```python
from build123d import *

# Parameters (mm, degrees)
SKIZZE1_W                       = 61.8
SKIZZE1_H                       = 93.64
AUFSATZ_LINEAR_AUSTRAGEN1_DEPTH = 6
VERRUNDUNG1_R                   = 6
WANDUNG1_T                      = -1
SKIZZE2_W                       = 21.5
SKIZZE2_H                       = 9.5
SCHNITT_LINEAR_AUSTRAGEN1_DEPTH = 6
SKIZZE3_W                       = 22
SKIZZE3_H                       = 5
SCHNITT_LINEAR_AUSTRAGEN2_DEPTH = 6
SCHNITT_LINEAR_AUSTRAGEN4_DEPTH = 6
LINEARES_MUSTER1_COUNT          = 3
LINEARES_MUSTER1_PITCH          = 25


with BuildPart() as part:
    # Skizze1 → Aufsatz-Linear austragen1 (new body)
    with BuildSketch(Plane(origin=(0, 0, 0), x_dir=(0, 1, 0), z_dir=(0, 0, 1))):
        Rectangle(SKIZZE1_W, SKIZZE1_H)
    extrude(amount=AUFSATZ_LINEAR_AUSTRAGEN1_DEPTH)

    # Verrundung1
    verrundung1_edges = [part.edges().sort_by_distance(p)[0] for p in [
        (46.82, 30.9, 3),
        (46.82, -30.9, 3),
        (-46.82, -30.9, 3),
        (-46.82, 30.9, 3),
    ]]
    fillet(verrundung1_edges, radius=VERRUNDUNG1_R)

    # Wandung1
    wandung1_openings = [part.faces().sort_by_distance(p)[0] for p in [
        (0, 0, 6),
    ]]
    offset(amount=WANDUNG1_T, openings=wandung1_openings, kind=Kind.INTERSECTION)

    # Skizze2 → Schnitt-Linear austragen1 (cut)
    with BuildSketch(Plane.YZ.offset(46.82)):
        with Locations((0, 6)):
            Rectangle(SKIZZE2_W, SKIZZE2_H)
    extrude(amount=-SCHNITT_LINEAR_AUSTRAGEN1_DEPTH, mode=Mode.SUBTRACT)

    # Skizze3 → Schnitt-Linear austragen2 (cut)
    with BuildSketch(Plane.XZ.offset(30.9)):
        with Locations((-11.18, 3.5)):
            Rectangle(SKIZZE3_W, SKIZZE3_H)
    extrude(amount=-SCHNITT_LINEAR_AUSTRAGEN2_DEPTH, mode=Mode.SUBTRACT)

    # Skizze4 → Schnitt-Linear austragen4 (cut)
    with BuildSketch(Plane(origin=(0, 0, 0), x_dir=(1, 0, 0), z_dir=(0, 0, -1))):
        Polygon((-25.159745962, 25.45), (-33.82, 20.45), (-33.82, 10.45), (-25.159745962, 5.45), (-16.499491924, 10.45), (-16.499491924, 20.45), align=None)
        Polygon((-25.159745962, -4.35), (-33.82, -9.35), (-33.82, -19.35), (-25.159745962, -24.35), (-16.499491924, -19.35), (-16.499491924, -9.35), align=None)
    schnitt_linear_austragen4 = extrude(amount=-SCHNITT_LINEAR_AUSTRAGEN4_DEPTH, mode=Mode.SUBTRACT)

    # Lineares Muster1: Schnitt-Linear austragen4 ×3
    with Locations(*[(i * LINEARES_MUSTER1_PITCH, 0, 0) for i in range(1, LINEARES_MUSTER1_COUNT)]):
        add(schnitt_linear_austragen4, mode=Mode.SUBTRACT)


solid = part.part
```
Can you work these out from the model? Positions are in its coordinate system, mm. A direction names the side the tool comes from. Coordinates: 2 decimals unless noted, no trailing zeros. Loops run counter-clockwise (first coordinate to the right, second up) from the corner with the lowest first, then second, coordinate; pieces in that order, holes last.
Item 1: Suppose I cut it at C-C (x = -19). Please give me the cut outline in (y, z).
Answers below:
outline: (-30.9, 0) - (-21.89, 0) - (-21.89, 1) - (-30.9, 1) - close; (-9.01, 0) - (7.91, 0) - (7.91, 1) - (-9.01, 1) - close; (20.79, 0) - (30.9, 0) - (30.9, 6) - (29.9, 6) - (29.9, 1) - (20.79, 1) - close
Item 2: If we mould it in two halves opening along Y, with no side actions, what happens to faces 1 (the face through (45.109, 29.096, 3.042)), 2 (the face through (-1, 0, 0)), 3 (the face through (-31, -29.9, 3))? For each: released by +Y, released by -Y, zero draft, split by the parting line, or undercut.
Answers below:
face 1: released by +Y
face 2: zero draft
face 3: undercut
Item 3: Suppose I cut it at B-B (z = 5). Please give me the cut outline in (x, y), then the cut area to 3 significant figures.
Answers below:
outline: (-46.82, -24.9) arc R6 ccw to (-40.82, -30.9) - (-22.18, -30.9) - (-22.18, -29.9) - (-40.82, -29.9) arc R5 cw to (-45.82, -24.9) - (-45.82, 24.9) arc R5 cw to (-40.82, 29.9) - (40.82, 29.9) arc R5 cw to (45.82, 24.9) - (45.82, 10.75) - (46.82, 10.75) - (46.82, 24.9) arc R6 ccw to (40.82, 30.9) - (-40.82, 30.9) arc R6 ccw to (-46.82, 24.9) - close; (-0.18, -30.9) - (40.82, -30.9) arc R6 ccw to (46.82, -24.9) - (46.82, -10.75) - (45.82, -10.75) - (45.82, -24.9) arc R5 cw to (40.82, -29.9) - (-0.18, -29.9) - close
area: 254 mm2
Item 4: Suppose I cut it at D-D (y = 1). Please give me the cut outline in (x, z), then the cut area to 3 significant figures.
Answers below:
outline: (-46.82, 0) - (46.82, 0) - (46.82, 1.25) - (45.82, 1.25) - (45.82, 1) - (-45.82, 1) - (-45.82, 6) - (-46.82, 6) - close
area: 98.9 mm2
Item 5: Which directions (+Z, -Z, +X, -X, +Y, -Y) give clear straight access to the entire face, cutting with the end or side of a thin tool? Please do faces 4 (the face through (29.231, 6.885, 0.493)), 5 (the face through (-44.32, -28.47, 3.54)), 6 (the face through (-46.82, 0, 3)).
Answers below:
face 4: +Z, -Z
face 5: +Z
face 6: +Z, -Z, -X, +Y, -Y
Item 6: I'm going to push flat-ended pins straight in: pin 1 (0.8 mm diameter, centred on x = 46.5, y = 1, fed in from +Z); pin 2 (6 mm diameter, centred on x = 37, y = -22, fed in from +Z); pin 3 (2.5 mm diameter, centred on y = -9, z = 3, fed in from +X). Where does each tip first touch, or does it pass through?
Answers below:
pin 1: stops at z = 1.25
pin 2: stops at z = 1
pin 3: stops at x = -45.82
Item 7: Suppose I cut it at A-A (y = 17). Please give me the cut outline in (x, z), then the cut area to 3 significant figures.
Answers below:
outline: (-46.82, 0) - (-33.82, 0) - (-33.82, 1) - (-45.82, 1) - (-45.82, 6) - (-46.82, 6) - close; (-16.5, 0) - (-8.82, 0) - (-8.82, 1) - (-16.5, 1) - close; (8.5, 0) - (16.18, 0) - (16.18, 1) - (8.5, 1) - close; (33.5, 0) - (46.82, 0) - (46.82, 6) - (45.82, 6) - (45.82, 1) - (33.5, 1) - close
area: 51.7 mm2
Item 8: Please list where these lines run through material, in increasing order: L1, parallel to X at y = 19, z = 4.2; L2, parallel to X at y = 24, z = 0.85; L3, parallel to X at y = 9, z = 0.95.
Answers below:
L1: x = -46.82 to -45.82, 45.82 to 46.82
L2: x = -46.82 to -25.77, -24.55 to -0.77, 0.45 to 24.23, 25.45 to 46.82
L3: x = -46.82 to -33.21, -17.11 to -8.21, 7.89 to 16.79, 32.89 to 46.82
